Here's how the part is built. I have some questions about the finished solid (model axes, mm). Round coordinates to 2 decimals unless told otherwise and drop trailing zeros. Write each loop counter-clockwise with the first axis right and the second up, starting at its lowest first coordinate (ties: lowest second). Pieces come first, ordered by that corner, then holes. Notation, with made-up numbers: (-21, -22.75) -> (-8, -22.75) arc R16 cw to (-8, -1.75) -> close; hole circle Ø8 at (14, 32). An arc over 180 degrees is marked (long way). Answer as CSV lines item,"result".
```python
from build123d import *

# Parameters (mm, degrees)
EXTRUDE1_DEPTH = 12.7
FILLET1_R      = 0.508


with BuildPart() as part:
    # Sketch1 → Extrude1 (new body, symmetric)
    with BuildSketch(Plane.XY):
        Polygon((0, 13.081), (0, 0), (13.081, 0), (13.081, 1.27), (1.27, 13.081), align=None)
    extrude(amount=EXTRUDE1_DEPTH, both=True)

    # Fillet1
    fillet1_edges = [part.edges().sort_by_distance(p)[0] for p in [
        (13.081, 0, 0),
        (0, 0, 0),
        (0, 13.081, 0),
    ]]
    fillet(fillet1_edges, radius=FILLET1_R)


solid = part.part
```
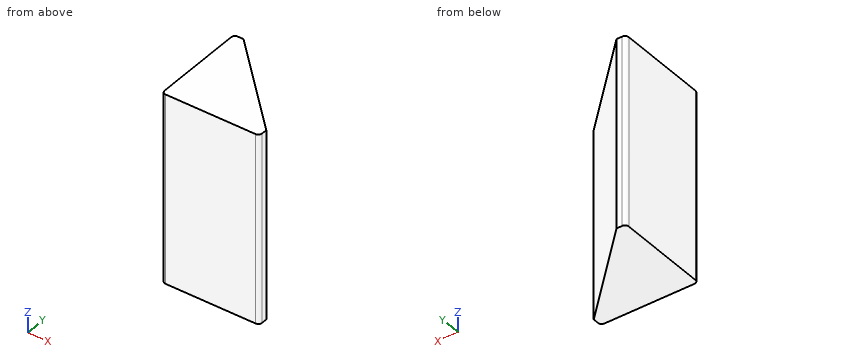
1. If I drill on line 1 (X direction, y = 11.5, z = -9.75); line 2 (Y direction, x = 10.5, z = -8.75); line 3 (X direction, y = 9.5, z = -7), over which ranges is the centre line in solid material (lowest first)?
Numbers:
line 1,"x = 0 to 2.85"
line 2,"y = 0 to 3.85"
line 3,"x = 0 to 4.85"
2. Suppose I cut it at A-A on z = -4.25. Please give me the cut outline in (x, y), and give its area (3 significant figures).
Numbers:
outline,"(0, 0.51) arc R0.51 ccw to (0.51, 0) -> (12.57, 0) arc R0.51 ccw to (13.08, 0.51) -> (13.08, 1.27) -> (1.27, 13.08) -> (0.51, 13.08) arc R0.51 ccw to (0, 12.57) -> close"
area,"101 mm^2"
3. Suppose I cut it at C-C on y = 6.75. Please give me the cut outline in (x, z).
Numbers:
outline,"(0, -12.7) -> (7.6, -12.7) -> (7.6, 12.7) -> (0, 12.7) -> close"
4. Suppose I cut it at B-B on x = 10. Please give me the cut outline in (y, z).
Numbers:
outline,"(0, -12.7) -> (4.35, -12.7) -> (4.35, 12.7) -> (0, 12.7) -> close"
5. For pin 1 Ø1.5 at (y, z) = (2.5, 9) entering from +X; pin 2 Ø1 at (x, y) = (9.5, 7) entering from -Z, each with a flat end and sliding along its axis, tell me the tip position at first contact or that it passes through.
Numbers:
pin 1,"stops at x = 12.6"
pin 2,"passes through"
